Design review of the part built by this model. Coordinates are the model's own, in mm. A direction names the side the tool comes from. Give positions to 0.01 mm unless a question says otherwise; leave off trailing zeros. Order: outer loops, then holes, each group sorted by start corner. A loop starts at its lowest first (then second) coordinate and runs counter-clockwise, first axis right, second up. Notation, with made-up numbers: (-13, 67) -> (-1, 67) arc R30 ccw to (-1, 106) -> close; hole circle Ø7 at (-22.75, 62.5). An arc over 180 degrees is marked (long way). Return JSON: item names as keys, results as strings.
```python
from build123d import *

# Parameters (mm, degrees)
CIRPATTERN1_COUNT = 4


with BuildPart() as part:
    # Sketch1 → Body (revolve)
    with BuildSketch(Plane.XY):
        Polygon((-12.7, -38.416258567), (-10.16, -38.416258567), (-3.884, -8.89), (-3.884, -6.35), (-6.985, 0), (-9.525, 0), (-9.525, -3.81), (-7.366, -3.81), (-7.366, -6.19125), (-9.525, -6.19125), (-9.525, -15.24), (-7.773734167, -15.24), align=None)
    revolve(axis=Axis((0, 0, 0), (0, -1, 0)))

    # Sketch4 → SetScrew (revolve, cut)
    with BuildSketch(Plane(origin=(-9.525, -10.63625, 0), x_dir=(0, 0, 1), z_dir=(0, 1, 0))):
        Polygon((0, 0), (0, 3.81), (2.45745, 2.333415072), (2.45745, 0), align=None)
    setscrew = revolve(axis=Axis((-15.875, -10.63625, 0), (1, 0, 0)), mode=Mode.SUBTRACT)

    # CirPattern1: SetScrew ×4 about axis
    cirpattern1_axis = Axis((0, 0, 0), (0, 1, 0))
    for i in range(1, CIRPATTERN1_COUNT):
        add(setscrew.rotate(cirpattern1_axis, i * 360 / CIRPATTERN1_COUNT), mode=Mode.SUBTRACT)


solid = part.part
```
Item 1: Wall thickness on L1, parallel to Z at x = 0, y = -7.9 (3 decimals); L2, parallel to X at y = -33, z = -7.25; L3, parallel to X at y = -35, z = 1.5: over which ranges is each line inside the solid? List them lowest first. Write a range as [from, to].
Result set:
{"L1": "z = [-9.525, -3.884], [3.884, 9.525]", "L2": "x = [-8.99, -5.35], [5.35, 8.99]", "L3": "x = [-11.88, -9.31], [9.31, 11.88]"}
Item 2: For pin 1 (6 mm diameter, centred on y = -4.5, z = -6, fed in from -X); pin 2 (4.5 mm diameter, centred on y = -10.64, z = 0, fed in from -X); pin 3 (10 mm diameter, centred on x = -5.5, y = -21, fed in from -Z), all flat-tipped, find the tip position at first contact; note any pin that passes through.
Result set:
{"pin 1": "stops at x = -9.01", "pin 2": "stops at x = -7.07", "pin 3": "stops at z = -9.55"}
Item 3: Add section A-A (y = -31). Give the boundary of the cut face in (x, z).
Result set:
{"outline": "circle Ø22.25 at (0, 0); hole circle Ø17.17 at (0, 0)"}
Item 4: Add section B-B (y = -20.5). Give the boundary of the cut face in (x, z).
Result set:
{"outline": "circle Ø17.78 at (0, 0); hole circle Ø12.7 at (0, 0)"}
Item 5: Mouldability with a two-part tool opening along Y and no side actions: class faces 5 (the face through (-5, -3.81, 6)), 6 (the face through (-6.656, -23.446, -2.096)), 7 (the face through (0.959, -5.247, 4.317)) as released by +Y, released by -Y, zero draft, split by the parting line, or undercut.
Result set:
{"face 5": "undercut", "face 6": "released by -Y", "face 7": "released by +Y"}
Item 6: Machinability: for faces 1 (the face through (-8.37, -9.7, 2.27)), 2 (the face through (8.37, -9.7, -2.27)), 3 (the face through (-3.399, -5.017, 6.535)), 4 (the face through (-8.8, -10.78, 3.65)), which of the approach directions +Z, -Z, +X, -X, +Y, -Y give a long, thin tool a straight path to every point of the face, cutting with its end or side? Answer none if there is none.
Result set:
{"face 1": "-X", "face 2": "+X", "face 3": "none", "face 4": "+Y"}
